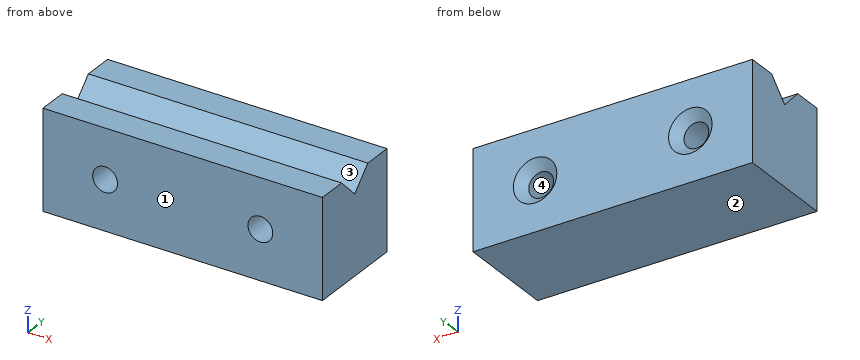
from build123d import *

# Parameters (mm, degrees)
BOSS_EXTRUDE1_DEPTH   = 45
F_1_0MM_DOWEL_HOLE1_D = 8
CHAMFER1_SIZE         = 3


with BuildPart() as part:
    # Sketch1 → Boss-Extrude1 (new, symmetric)
    with BuildSketch(Plane(origin=(0, 0, 0), x_dir=(0, 0, -1), z_dir=(1, 0, 0))):
        Polygon((-16, 16), (-16, 6.5), (-9.5, 0), (-16, -6.5), (-16, -16), (16, -16), (16, 16), align=None)
    extrude(amount=BOSS_EXTRUDE1_DEPTH, both=True)

    # Ø1.0mm Dowel Hole1 (through all)
    with Locations(Plane(origin=(0, 16, 0), x_dir=(1, 0, 0), z_dir=(0, 1, 0))):
        with Locations((25, 0), (-25, 0)):
            Hole(F_1_0MM_DOWEL_HOLE1_D / 2)

    # Chamfer1
    chamfer1_edges = [part.edges().sort_by_distance(p)[0] for p in [
        (-21, 16, 0),
        (29, 16, 0),
    ]]
    chamfer(chamfer1_edges, length=CHAMFER1_SIZE)


solid = part.part
Could you check a few things on this model? Use its own coordinates, in mm. Face numbers are marked on the shaded views. Give positions to 0.01 mm unless a question says otherwise; leave off trailing zeros. Write each loop counter-clockwise with the first axis right and the second up, starting at its lowest first coordinate (ties: lowest second). Pieces come first, ordered by that corner, then holes. Notation, with made-up numbers: (49.25, -2) -> (83.25, -2) arc R22 cw to (83.25, 28) -> close; hole circle Ø6 at (50.5, -4). An arc over 180 degrees is marked (long way). Write each question's results on one line, items separated by ' | '. Start each with the question number.
Q1. We'd pull the mould along Z, two halves only. Please class the marked faces 1, 2, 3 and 4: +Z half, -Z half, draft (parallel to the pull), parting line (faces both ways), or undercut.
Q2. Suppose I cut it at A-A, the plane x = -25. List the corners of the cut face in (y, z) for me.
Q3. Suppose I cut it at B-B, the plane z = 0. List the corners of the cut face in (x, y) for me.
Q4. I need wall thicknesses on probe 1 along X at (y, z) = (-1.5, 0); probe 2 along Z at (x, y) = (-25, 0); probe 3 along X at (y, z) = (-5, -3). Which ranges of each line are inside material? Lowest first, please.
Q5. I'm going to push flat-ended pins straight in: pin 1 Ø9 at (x, z) = (25, 0) entering from +Y; pin 2 Ø12 at (x, y) = (-25.5, -4) entering from +Z; pin 3 Ø4 at (x, y) = (-35.5, -2) entering from +Z; pin 4 Ø4 at (x, y) = (4, 0) entering from +Z. Where does each tip first touch, or does it pass through?
Q6. Suppose I cut it at D-D, the plane z = 14.5. List the corners of the cut face in (x, y) for me.
Q7. Suppose I cut it at C-C, the plane y = 3. List the corners of the cut face in (x, z) for me.
Outcome:
1) face 1: draft | face 2: -Z half | face 3: +Z half | face 4: undercut
2) outline: (-16, -16) -> (16, -16) -> (16, -7) -> (13, -4) -> (-16, -4) -> close; (-16, 4) -> (13, 4) -> (16, 7) -> (16, 16) -> (6.5, 16) -> (0, 9.5) -> (-6.5, 16) -> (-16, 16) -> close
3) outline: (-45, -16) -> (-29, -16) -> (-29, 13) -> (-32, 16) -> (-45, 16) -> close; (-21, -16) -> (21, -16) -> (21, 13) -> (18, 16) -> (-18, 16) -> (-21, 13) -> close; (29, -16) -> (45, -16) -> (45, 16) -> (32, 16) -> (29, 13) -> close
4) probe 1: -45 to -29, -21 to 21, 29 to 45 | probe 2: -16 to -4, 4 to 9.5 | probe 3: -45 to -27.65, -22.35 to 22.35, 27.65 to 45
5) pin 1: y = 13.5 | pin 2: z = 16 | pin 3: z = 13.5 | pin 4: z = 11.5
6) outline: (-45, -16) -> (45, -16) -> (45, -5) -> (-45, -5) -> close; (-45, 5) -> (45, 5) -> (45, 16) -> (-45, 16) -> close
7) outline: (-45, -16) -> (45, -16) -> (45, 12.5) -> (-45, 12.5) -> close; hole circle Ø8 at (-25, 0); hole circle Ø8 at (25, 0)
